Build history of the part. All positions in model axes, mm. A direction names the side the tool comes from. Give positions to 0.01 mm unless a question says otherwise; leave off trailing zeros. Loops run counter-clockwise (first coordinate to the right, second up) from the corner with the lowest first, then second, coordinate; pieces in that order, holes last. Notation, with made-up numbers: (82.25, 79.25) -> (136.25, 79.25) arc R14 cw to (136.25, 89.25) -> close; hole circle Ø3 at (60.25, 85.25). An arc over 180 degrees is marked (long way). One line per question, with ' | ' between items. Start each with the question number.
(1) Slice it at D-D, the plane y = 11. Write the cut outline in (x, z), then the cut area to 3 significant figures.
(2) Drill centre lines: L1, parallel to Y at x = 0.75, z = -3.75; L2, parallel to Y at x = 0.5, z = -2.75; L3, parallel to Y at x = -2.5, z = 4.5. Where is each one in solid material? Low to high. Write a range as from..to.
(3) Slice it at C-C, the plane y = -19. Write the cut outline in (x, z).
(4) 3-axis set-ups, long thin cutter, end or side, ignore diameter. For faces 1 (the face through (-5.303, 0, 1)), 2 (the face through (-1.985, 10.483, -2.134)): which of +Z, -Z, +X, -X, +Y, -Y reach the whole face in a straight line?
(5) Flat gauge pin, fed straight in: pin 1 Ø4 at (x, z) = (0.5, -3) entering from -Y. Where does the tip first touch, or does it go through?
(6) Slice it at B-B, the plane z = 2.25. Write the cut outline in (x, y).
(7) Slice it at A-A, the plane x = 4.5. Write the cut outline in (y, z), then the cut area to 3 significant figures.
```python
from build123d import *

# Parameters (mm, degrees)
F0_W     = 10.6066017178
F0_H     = 10.6066017178
F1_DEPTH = 22.5
F4_DEPTH = 15
F6_DEPTH = 15
F8_DEPTH = 15


# Not quite as in the source:
# - a feature names something its author has since deleted; it is built from what else it names


with BuildPart() as f1:
    # F0 (on Front) → F1 (new body, symmetric)
    with BuildSketch(Plane.XZ):
        Rectangle(F0_W, F0_H)
    extrude(amount=F1_DEPTH, both=True)

    # F3 (on 3pt) → F4 (cut, symmetric)
    with BuildSketch(Plane(origin=(0, 0, 0), x_dir=(0, 1, 0), z_dir=(0.7071067812, 0, -0.7071067812))):
        Polygon((-15, -7.5), (-22.5, 0), (-15, 7.5), (-15, 9.5), (-24.5, 9.5), (-24.5, -9.5), (-15, -9.5), align=None)
        Polygon((15, 7.5), (22.5, 0), (15, -7.5), (15, -9.5), (24.5, -9.5), (24.5, 9.5), (15, 9.5), align=None)
    extrude(amount=F4_DEPTH, both=True, mode=Mode.SUBTRACT)

    # F5 (on 3pt) → F6 (cut, symmetric)
    with BuildSketch(Plane(origin=(0, 0, 0), x_dir=(0, 1, 0), z_dir=(0.7071067812, 0, -0.7071067812))):
        Polygon((7.5, 0), (0, -7.5), (-7.5, 0), (-15, -7.5), (-15, -9.5), (15, -9.5), (15, -7.5), align=None)
    extrude(amount=F6_DEPTH, both=True, mode=Mode.SUBTRACT)

    # F7 (on 3pt) → F8 (cut, symmetric)
    with BuildSketch(Plane(origin=(0, 0, 0), x_dir=(0, 1, 0), z_dir=(0.7071067812, 0, -0.7071067812))):
        Polygon((-7.5, 0.0707106781), (-16.0707106781, -8.5), (16.0707106781, -8.5), (7.5, 0.0707106781), (0, -7.4292893219), align=None)
    extrude(amount=F8_DEPTH, both=True, mode=Mode.SUBTRACT)


solid = f1.part
```
Final values:
1) outline: (-5.3, 0.45) -> (0.45, -5.3) -> (5.3, -5.3) -> (5.3, 5.3) -> (-5.3, 5.3) -> close | area: 95.9 mm2
2) L1: -20.38..-9.69, -5.31..5.31, 9.69..20.38 | L2: -20.91..-9.16, -5.84..5.84, 9.16..20.91 | L3: -21.09..21.09
3) outline: (-5.3, 0.35) -> (0.35, -5.3) -> (5.3, -5.3) -> (5.3, -0.35) -> (-0.35, 5.3) -> (-5.3, 5.3) -> close
4) face 1: +Z, -Z, -X, +Y, -Y | face 2: -Z, -X
5) pin 1: y = -22.5
6) outline: (-5.3, -20.34) -> (-2.25, -22.5) -> (5.3, -17.16) -> (5.3, 17.16) -> (-2.25, 22.5) -> (-5.3, 20.34) -> (-5.3, 9.73) -> (-2.15, 7.5) -> (-5.3, 5.27) -> (-5.3, -5.27) -> (-2.15, -7.5) -> (-5.3, -9.73) -> close
7) outline: (-22.5, -4.5) -> (-21.93, -5.3) -> (-8.14, -5.3) -> (-7.5, -4.4) -> (-6.86, -5.3) -> (6.86, -5.3) -> (7.5, -4.4) -> (8.14, -5.3) -> (21.93, -5.3) -> (22.5, -4.5) -> (15.57, 5.3) -> (-15.57, 5.3) -> close | area: 408 mm2
